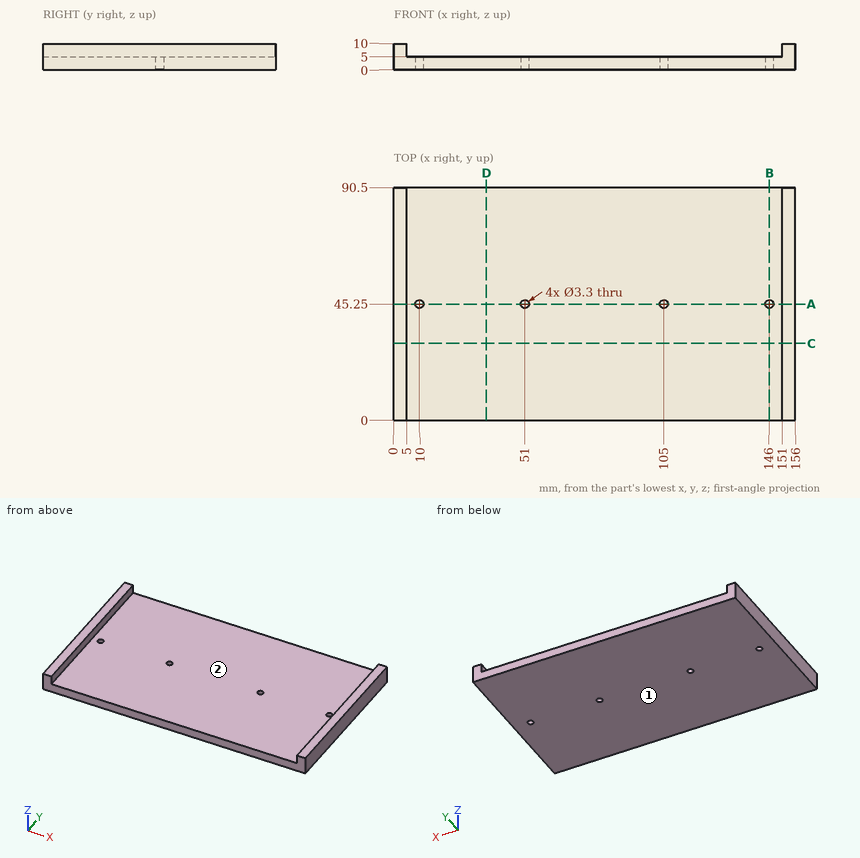
Study the drawing (mm; zero at the part's minimum x, y, z) and answer. Coordinates: 2 decimals unless noted, no trailing zeros. Write each loop counter-clockwise with the first axis right and the second up, starting at its lowest first coordinate (ties: lowest second). Pieces come first, ordered by that corner, then holes. Notation, with made-up numbers: (59, 43.5) - (98, 43.5) arc R31 ccw to (98, 67.5) - close; hole circle Ø8 at (21, 43). An arc over 180 degrees is marked (long way). Return JSON: item names as keys, results as strings. Group by question number.
1. A cutting plane is placed at A-A, the plane y = 45.25. Determine the outline of the cut face in (x, z), plus the area to 3 significant figures.
2. Straight lines are drawn through the part: L1, parallel to X at y = 45.25, z = 1.2; L2, parallel to X at y = 83, z = 6.75; L3, parallel to Y at x = 10, z = 3.95. For each, find the intervals that lie inside material, in ascending order.
3. A cutting plane is placed at C-C, the plane y = 30. Determine the outline of the cut face in (x, z), plus the area to 3 significant figures.
4. Given pin 1 (8 mm diameter, centred on x = 24.5, y = 79.5, fed in from +Z); pin 2 (3 mm diameter, centred on x = 146, y = 45.25, fed in from -Z), each flat-ended and moving along its own axis, determine where each tip first touches the part or whether it passes through.
5. Determine the mould class of the marked faces 1 and 2 for opening direction X: released by +X, released by -X, zero draft, split by the parting line, or undercut.
6. A cutting plane is placed at D-D, the plane x = 36. Determine the outline of the cut face in (y, z).
7. A cutting plane is placed at B-B, the plane x = 146. Determine the outline of the cut face in (y, z), plus the area to 3 significant figures.
Ans:
{
 "1": {"outline": "(0, 0) - (8.35, 0) - (8.35, 5) - (5, 5) - (5, 10) - (0, 10) - close; (11.65, 0) - (49.35, 0) - (49.35, 5) - (11.65, 5) - close; (52.65, 0) - (103.35, 0) - (103.35, 5) - (52.65, 5) - close; (106.65, 0) - (144.35, 0) - (144.35, 5) - (106.65, 5) - close; (147.65, 0) - (156, 0) - (156, 10) - (151, 10) - (151, 5) - (147.65, 5) - close", "area": "764 mm²"},
 "2": {"L1": "0 to 8.35, 11.65 to 49.35, 52.65 to 103.35, 106.65 to 144.35, 147.65 to 156", "L2": "0 to 5, 151 to 156", "L3": "0 to 43.6, 46.9 to 90.5"},
 "3": {"outline": "(0, 0) - (156, 0) - (156, 10) - (151, 10) - (151, 5) - (5, 5) - (5, 10) - (0, 10) - close", "area": "830 mm²"},
 "4": {"pin 1": "z = 5", "pin 2": "through"},
 "5": {"face 1": "zero draft", "face 2": "undercut"},
 "6": {"outline": "(0, 0) - (90.5, 0) - (90.5, 5) - (0, 5) - close"},
 "7": {"outline": "(0, 0) - (43.6, 0) - (43.6, 5) - (0, 5) - close; (46.9, 0) - (90.5, 0) - (90.5, 5) - (46.9, 5) - close", "area": "436 mm²"}
}
